The listing builds one solid part. Answer for the finished solid, in the listing's coordinates (mm). A direction names the side the tool comes from. Give positions to 0.01 mm unless a question says otherwise; leave off trailing zeros. Order: outer loops, then holes, each group sorted by start corner. A loop starts at its lowest first (then second) coordinate and runs counter-clockwise, first axis right, second up. Notation, with made-up numbers: (7, 45.25) - (42, 45.25) arc R18 cw to (42, 49.25) - close; hole circle Ø7 at (67.5, 37). An arc over 180 degrees is marked (long way). Use a Markdown table: item, result. Add a question column.
1) The mould has two halves that part along X. Classify faces 1 (the face through (116.92, -116.56, 5.07)), 2 (the face through (137.5, -2, 5)), 3 (the face through (-111.94, 111.62, 12.98)), 4 (the face through (-128.479, 128.945, 4.93)): released by +X, released by -X, zero draft, split by the parting line, or undercut.
2) For faces 5 (the face through (132.4, -1.5, 15.1)), 6 (the face through (-108.08, 108.44, 5.07)), determine the directions among +Z, -Z, +X, -X, +Y, -Y from which every point of the face is accessible in a straight line to the end or side of a thin tool.
3) Straight lines are drawn through the part: line 1 (Y direction, x = -112.5, z = 4.75); line 2 (Y direction, x = 114, z = 7). For each, find the intervals that lie inside material, in ascending order.
4) Flat-ended cylindrical pins translate along their axes: pin 1 (1 mm diameter, centred on y = 67, z = 12.5, fed in from +X); pin 2 (11 mm diameter, centred on x = 112.5, y = 112.5, fed in from -Z); pin 3 (1.5 mm diameter, centred on y = 90.5, z = 15, fed in from -X). Find the tip coordinate at first contact, or state that the pin passes through.
5) Find section A-A, the plane z = 16.75. Determine the outline of the cut face in (x, y), plus the area to 3 significant figures.
6) Find section B-B, the plane y = 38. Determine the outline of the cut face in (x, z).
from build123d import *

# Parameters (mm, degrees)
F1_DEPTH = 20
F2_SIZE  = 10
F4_D     = 12
F4_DEPTH = 10
F4_TIP   = 3.6051637142


with BuildPart() as f1:
    # F0 (on Top) → F1 (new body)
    with BuildSketch(Plane.XY):
        with BuildLine():
            Line((107.5, 137.5), (-107.5, 137.5))
            ThreePointArc((-107.5, 137.5), (-128.7132034356, 128.7132034356), (-137.5, 107.5))
            Line((-137.5, 107.5), (-137.5, -107.5))
            ThreePointArc((-137.5, -107.5), (-128.7132034356, -128.7132034356), (-107.5, -137.5))
            Line((-107.5, -137.5), (107.5, -137.5))
            ThreePointArc((107.5, -137.5), (128.7132034356, -128.7132034356), (137.5, -107.5))
            Line((137.5, -107.5), (137.5, 107.5))
            ThreePointArc((137.5, 107.5), (128.7132034356, 128.7132034356), (107.5, 137.5))
        make_face()
    extrude(amount=F1_DEPTH)

    # F2
    f2_edges = [f1.edges().sort_by_distance(p)[0] for p in [
        (-137.5, 0, 20),
    ]]
    chamfer(f2_edges, length=F2_SIZE)

    # F4
    with Locations(Plane(origin=(0, 0, 0), x_dir=(1, 0, 0), z_dir=(0, 0, -1))):
        with Locations((-112.5, 112.5), (112.5, 112.5), (112.5, -112.5), (-112.5, -112.5)):
            Hole(F4_D / 2, depth=F4_DEPTH)
            with Locations((0, 0, -(F4_DEPTH + F4_TIP / 2))):  # 118° drill point
                Cone(0, F4_D / 2, F4_TIP, mode=Mode.SUBTRACT)


solid = f1.part
The answers:
| question | item | result |
|---|---|---|
| 1 | face 1 | undercut |
| 1 | face 2 | released by +X |
| 1 | face 3 | undercut |
| 1 | face 4 | released by -X |
| 2 | face 5 | +Z, +X, +Y, -Y |
| 2 | face 6 | -Z |
| 3 | line 1 | -137.08 to -118.5, -106.5 to 106.5, 118.5 to 137.08 |
| 3 | line 2 | -136.79 to -118.31, -106.69 to 106.69, 118.31 to 136.79 |
| 4 | pin 1 | x = 135.5 |
| 4 | pin 2 | z = 10.3 |
| 4 | pin 3 | x = -133.25 |
| 5 | outline | (-130.75, -107.5) arc R23.25 ccw to (-107.5, -130.75) - (107.5, -130.75) arc R23.25 ccw to (130.75, -107.5) - (130.75, 107.5) arc R23.25 ccw to (107.5, 130.75) - (-107.5, 130.75) arc R23.25 ccw to (-130.75, 107.5) - close |
| 5 | area | 67,900 mm2 |
| 6 | outline | (-137.5, 0) - (137.5, 0) - (137.5, 10) - (127.5, 20) - (-127.5, 20) - (-137.5, 10) - close |
